Geometry check sheet. Reference: drawing and pictorial views, mm from the part's lowest x, y, z. A direction names the side the tool comes from. Give positions to 0.01 mm unless a question says otherwise; leave off trailing zeros. Loops run counter-clockwise (first coordinate to the right, second up) from the corner with the lowest first, then second, coordinate; pieces in that order, holes last. Notation, with made-up numbers: (3.25, -36.75) -> (25.25, -36.75) arc R26 ccw to (25.25, -8.75) -> close; hole circle Ø6 at (41, 36.25). An arc over 180 degrees is marked (long way). Write item = value, one per line. Start each with the question number.
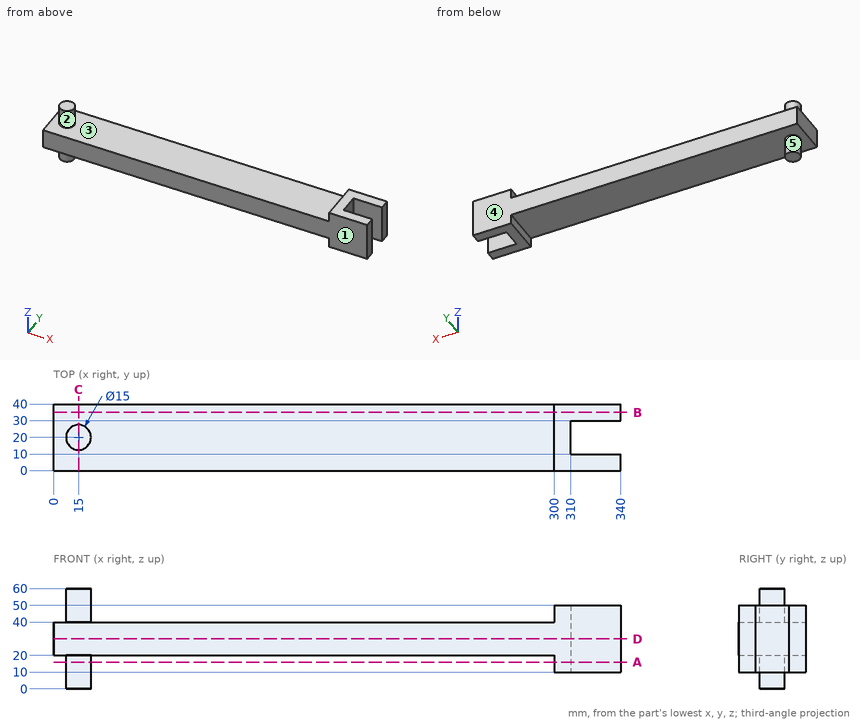
1) Draft check along X on the marked faces 3, 4 and 5. Enter one of: released by +X, released by -X, zero draft, split by the parting line, or undercut.
2) Section check C-C (x = 15). Enter the section's corners in (y, z), plus the area to 3 significant figures.
3) Section check A-A (z = 16). Enter the section's corners in (x, y), plus the area to 3 significant figures.
4) Thickness scan on line 1 (X direction, y = 14, z = 26.5); line 2 (Z direction, x = 174.5, y = 26); line 3 (X direction, y = 28, z = 13.5). Record the ranges inside material, lowest first.
5) Tool access check on the marked faces 1 and 2. Record the directions out of +Z, -Z, +X, -X, +Y, -Y that give a thin tool (end or side, any length) a straight path to the whole face; none if there is none.
6) Section check B-B (y = 35). Enter the section's corners in (x, z).
7) Section check D-D (z = 30). Enter the section's corners in (x, y), plus the area to 3 significant figures.
8) Depth check by flat-ended pin: pin 1 Ø20 at (x, y) = (223, 20.5) entering from +Z; pin 2 Ø12 at (x, y) = (279.5, 18.5) entering from -Z; pin 3 Ø10 at (y, z) = (11, 34) entering from -X; pin 4 Ø20 at (x, y) = (310.5, 17.5) entering from -Z. Enter the tip coordinate at first touch or a pass-through.
Check result:
q1.face_3 = undercut
q1.face_4 = zero draft
q1.face_5 = undercut
q2.outline = (0, 20) -> (12.5, 20) -> (12.5, 0) -> (27.5, 0) -> (27.5, 20) -> (40, 20) -> (40, 40) -> (27.5, 40) -> (27.5, 60) -> (12.5, 60) -> (12.5, 40) -> (0, 40) -> close
q2.area = 1,400 mm2
q3.outline = circle Ø15 at (15, 20); (300, 0) -> (340, 0) -> (340, 10) -> (310, 10) -> (310, 30) -> (340, 30) -> (340, 40) -> (300, 40) -> close
q3.area = 1,180 mm2
q4.line_1 = 0 to 310
q4.line_2 = 20 to 40
q4.line_3 = 300 to 310
q5.face_1 = +Z, -Z, +X, -X, -Y
q5.face_2 = +Z
q6.outline = (0, 20) -> (300, 20) -> (300, 10) -> (340, 10) -> (340, 50) -> (300, 50) -> (300, 40) -> (0, 40) -> close
q7.outline = (0, 0) -> (340, 0) -> (340, 10) -> (310, 10) -> (310, 30) -> (340, 30) -> (340, 40) -> (0, 40) -> close
q7.area = 13,000 mm2
q8.pin_1 = 40
q8.pin_2 = 20
q8.pin_3 = 0
q8.pin_4 = 10
